from build123d import *

# Parameters (mm, degrees)
SKETCH_1_W          = 16
SKETCH_1_H          = 38
EXTRUDE_1_DEPTH     = 4.6
CUT_EXTRUDE_3_REACH = 38.941
SKETCH_6_W          = 11.7
SKETCH_6_H          = 4.05
SKETCH_6_R          = 1
EXTRUDE_2_DEPTH     = 3.75
SKETCH_9_R          = 2.56
SKETCH_9_R_2        = 1.525
EXTRUDE_3_DEPTH     = 3
SKETCH_10_R         = 1.45
CUT_EXTRUDE_5_DEPTH = 2.5


with BuildPart() as part:
    # 草图1 → 凸台-拉伸1 (new body)
    with BuildSketch(Plane(origin=(-0.735865771, -2.984459331, 108.825789607), x_dir=(0.9999771565250809, -0.00018529520807729263, 0.006756633311043236), z_dir=(-0.006759173619166435, -0.027413258740008984, 0.9996013339413065))):
        with Locations((-12.117906651, 11.494673284)):
            Rectangle(SKETCH_1_W, SKETCH_1_H)
    extrude(amount=EXTRUDE_1_DEPTH)

    # 草图5 → 切除-拉伸3 (cut, up to next)
    with BuildSketch(Plane(origin=(-0.735865771, -2.984459331, 108.825789607), x_dir=(-0.9999771565250809, 0.0001852952080772962, -0.006756633311043381), z_dir=(0.00675917361916658, 0.02741325874000909, -0.9996013339413065)), mode=Mode.PRIVATE) as cut_extrude_3_sk1:
        with BuildLine():
            ThreePointArc((15.703441088, 8.166291382), (12.117906651, 13.014673284), (8.532372214, 8.166291382))
            ThreePointArc((8.532372214, 8.166291382), (12.117906651, -3.755326716), (15.703441088, 8.166291382))
        make_face()
    cut_extrude_3_tool1 = extrude(cut_extrude_3_sk1.sketch, amount=-CUT_EXTRUDE_3_REACH, mode=Mode.PRIVATE) & part.part
    add(cut_extrude_3_tool1.solids().sort_by_distance((-12.853496, 1.00994, 108.853395))[0], mode=Mode.SUBTRACT)

    # 草图6 → 凸台-拉伸2 (add)
    # profile 1 of 2: a face of its own
    with BuildSketch(Plane(origin=(-0.735865771, -2.984459331, 108.825789607), x_dir=(-0.9999771565250809, 0.0001852952080772936, -0.0067566333110433766), z_dir=(0.006759173619166576, 0.02741325874000879, -0.9996013339413065))):
        with Locations((12.117906651, 22.369673284)):
            Rectangle(SKETCH_6_W, SKETCH_6_H)
        with Locations(Location((12.117906651, 21.944673284, 0), (0, 0, 270))):
            Circle(SKETCH_6_R, mode=Mode.SUBTRACT)
    # profile 2 of 2: a face of its own
    with BuildSketch(Plane(origin=(-0.735865771, -2.984459331, 108.825789607), x_dir=(-0.9999771565250809, 0.0001852952080772936, -0.0067566333110433766), z_dir=(0.006759173619166576, 0.02741325874000879, -0.9996013339413065))):
        Polygon((7.267906651, -3.455326716), (17.967906651, -3.455326716), (17.967906651, -7.505326716), (6.267906651, -7.505326716), (6.267906651, -3.455326716), align=None)
        with Locations(Location((12.117906651, -5.055326716, 0), (0, 0, 270))):
            Circle(SKETCH_6_R, mode=Mode.SUBTRACT)
    extrude(amount=EXTRUDE_2_DEPTH)

    # 草图9 → 凸台-拉伸3 (add)
    with BuildSketch(Plane(origin=(-0.76695797, -3.110560321, 113.423955744), x_dir=(0.9999771565250809, -0.00018529520807729366, 0.006756633311043378), z_dir=(-0.006759173619166578, -0.02741325874000878, 0.9996013339413065))):
        with Locations(Location((-12.117906651, 25.004673284, 0), (0, 0, 90))):
            Circle(SKETCH_9_R)
        with Locations(Location((-12.117906651, 25.004673284, 0), (0, 0, 90))):
            Circle(SKETCH_9_R_2, mode=Mode.SUBTRACT)
    extrude(amount=EXTRUDE_3_DEPTH)

    # 草图10 → 切除-拉伸5 (cut)
    with BuildSketch(Plane(origin=(-0.76695797, -3.110560321, 113.423955744), x_dir=(0.9999771565250809, -0.00018529520807729366, 0.006756633311043378), z_dir=(-0.006759173619166578, -0.02741325874000879, 0.9996013339413065))):
        with Locations(Location((-12.117906651, 25.004673284, 0), (0, 0, 270))):
            Circle(SKETCH_10_R)
    extrude(amount=-CUT_EXTRUDE_5_DEPTH, mode=Mode.SUBTRACT)


solid = part.part
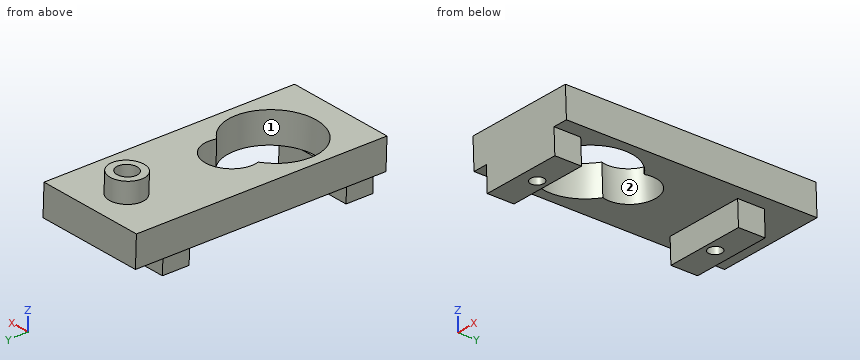
The listing builds one solid part. Answer for the finished solid, in the listing's coordinates (mm). Face numbers are marked on the shaded views. Round coordinates to 2 decimals unless told otherwise and drop trailing zeros. Order: outer loops, then holes, each group sorted by start corner. A loop starts at its lowest first (then second) coordinate and runs counter-clockwise, first axis right, second up. Notation, with made-up numbers: (12.5, -3) - (51.5, -3) arc R14 cw to (51.5, 21) - close; hole circle Ø11 at (75, 11). An arc over 180 degrees is marked (long way). Write item = value, one per line. Start each with the question number.
1) For a pull along Y with two mould halves and no side action, classify the marked faces 1 and 2 as released by +Y, released by -Y, zero draft, split by the parting line, or undercut.
2) Given pin 1 (5 mm diameter, centred on x = -17.5, z = 115.5, fed in from -Y); pin 2 (5 mm diameter, centred on x = -10.5, z = 108.5, fed in from +Y); pin 3 (1 mm diameter, centred on x = -10.5, y = 17, fed in from -Z); pin 4 (3 mm diameter, centred on x = -15, y = 4.5, fed in from -Z), each flat-ended and moving along its own axis, determine where each tip first touches the part or whether it passes through.
3) Straight lines are drawn through the part: L1, parallel to X at y = -8, z = 108; L2, parallel to Y at x = -12, z = 116.25; L3, parallel to X at y = 21.5, z = 115.25. For each, find the intervals that lie inside material, in ascending order.
4) Section A-A, the plane y = 25 is taken. Write down the section's boundary in (x, z).
Results list:
q1.face_1 = undercut
q1.face_2 = undercut
q2.pin_1 = -10.61
q2.pin_2 = 27.5
q2.pin_3 = 105.57
q2.pin_4 = through
q3.L1 = -18.7 to -13.85, -11.85 to -7
q3.L2 = 19.43 to 20.59, 23.06 to 24.22
q3.L3 = -15.43 to -14.38, -11.41 to -10.36
q4.outline = (-20.88, 114.06) - (-20.85, 109.46) - (-4.85, 109.57) - (-4.88, 114.17) - close
